```python
from build123d import *

# Parameters (mm, degrees)
SCHIZZO1_W                   = 570
SCHIZZO1_H                   = 450
ESTRUSIONE_ESTRUSIONE1_DEPTH = 10
SCHIZZO2_R                   = 2.25
SCHIZZO2_W                   = 23
SCHIZZO2_H                   = 20
SCHIZZO2_W_2                 = 20
SCHIZZO2_H_2                 = 23
TAGLIO_ESTRUSIONE1_DEPTH     = 10


with BuildPart() as part:
    # Schizzo1 → Estrusione-Estrusione1 (new body)
    with BuildSketch(Plane(origin=(0, 0, 0), x_dir=(1, 0, 0), z_dir=(0, 1, 0))):
        with Locations((-285, 225)):
            Rectangle(SCHIZZO1_W, SCHIZZO1_H)
    extrude(amount=ESTRUSIONE_ESTRUSIONE1_DEPTH)

    # Schizzo2 → Taglio-Estrusione1 (cut)
    with BuildSketch(Plane.XZ):
        with Locations(Location((-467, -68, 0), (0, 0, 270))):
            Circle(SCHIZZO2_R)
        with Locations(Location((-448.5, -68, 0), (0, 0, 270))):
            Circle(SCHIZZO2_R)
        with Locations(Location((-121.5, -68, 0), (0, 0, 270))):
            Circle(SCHIZZO2_R)
        with Locations(Location((-103, -68, 0), (0, 0, 270))):
            Circle(SCHIZZO2_R)
        with Locations(Location((-467, -382, 0), (0, 0, 270))):
            Circle(SCHIZZO2_R)
        with Locations(Location((-448.5, -382, 0), (0, 0, 270))):
            Circle(SCHIZZO2_R)
        with Locations(Location((-121.5, -382, 0), (0, 0, 270))):
            Circle(SCHIZZO2_R)
        with Locations(Location((-103, -382, 0), (0, 0, 270))):
            Circle(SCHIZZO2_R)
        with Locations(Location((-472, -420, 0), (0, 0, 270))):
            Circle(SCHIZZO2_R)
        with Locations(Location((-540, -352, 0), (0, 0, 270))):
            Circle(SCHIZZO2_R)
        with Locations(Location((-540, -98, 0), (0, 0, 270))):
            Circle(SCHIZZO2_R)
        with Locations(Location((-472, -30, 0), (0, 0, 270))):
            Circle(SCHIZZO2_R)
        with Locations(Location((-98, -30, 0), (0, 0, 270))):
            Circle(SCHIZZO2_R)
        with Locations(Location((-30, -98, 0), (0, 0, 270))):
            Circle(SCHIZZO2_R)
        with Locations(Location((-30, -352, 0), (0, 0, 270))):
            Circle(SCHIZZO2_R)
        with Locations(Location((-98, -420, 0), (0, 0, 270))):
            Circle(SCHIZZO2_R)
        with Locations((-472, -10)):
            Rectangle(SCHIZZO2_W, SCHIZZO2_H)
        with Locations((-98, -10)):
            Rectangle(SCHIZZO2_W, SCHIZZO2_H)
        with Locations((-10, -98)):
            Rectangle(SCHIZZO2_W_2, SCHIZZO2_H_2)
        with Locations((-10, -352)):
            Rectangle(SCHIZZO2_W_2, SCHIZZO2_H_2)
        with Locations((-98, -440)):
            Rectangle(SCHIZZO2_W, SCHIZZO2_H)
        with Locations((-472, -440)):
            Rectangle(SCHIZZO2_W, SCHIZZO2_H)
        with Locations((-560, -352)):
            Rectangle(SCHIZZO2_W_2, SCHIZZO2_H_2)
        with Locations((-560, -98)):
            Rectangle(SCHIZZO2_W_2, SCHIZZO2_H_2)
    extrude(amount=-TAGLIO_ESTRUSIONE1_DEPTH, mode=Mode.SUBTRACT)


solid = part.part
```
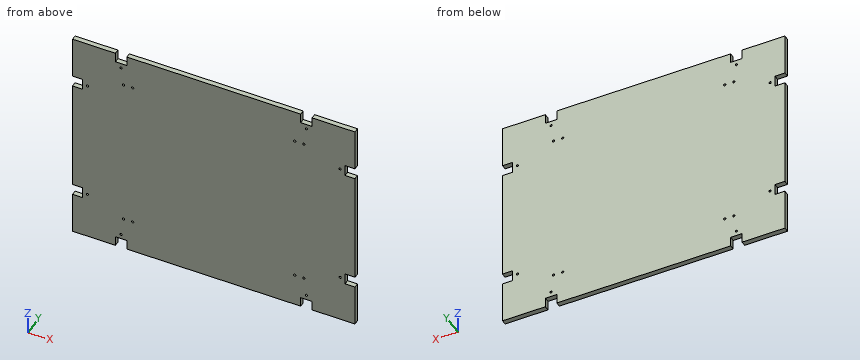
Read the model definition and answer for the solid it produces. Units are mm, in the model's axes. Round coordinates to 2 decimals unless told otherwise and drop trailing zeros. One line per item, written item: value.
Q1. Each of these flat-tipped pins is pushed along its axis until it touches: P1, Ø2.5, axis at x = -98, z = -420, coming from the +Y side; P2, Ø5, axis at x = -474, y = 6.5, coming from the +Z side. Where does it stop, or does it pass through?
The answers:
P1: passes through
P2: stops at z = -20
Q2. Straight lines are drawn through the part: line 1 (Z direction, x = -540, y = 6); line 2 (X direction, y = 6.25, z = -98); line 3 (X direction, y = 5, z = -420). For each, find the intervals that lie inside material, in ascending order. Write a range as from..to.
The answers:
line 1: z = -450..-354.25, -349.75..-100.25, -95.75..0
line 2: x = -550..-542.25, -537.75..-32.25, -27.75..-20
line 3: x = -570..-474.25, -469.75..-100.25, -95.75..0
Q3. Find section A-A (y = 5). Count the separate pieces of the cut face and the enclosed holes in it, and give its area (3 significant figures).
The answers:
separate pieces: 1
enclosed holes: 16
area: 253,000 mm2
